from build123d import *

# Parameters (mm, degrees)
SKETCH_W      = 80
SKETCH_H      = 150
PAD_DEPTH     = 2
FILLET_R      = 10
SKETCH001_R   = 19.147904
SKETCH001_R_2 = 1.5
POCKET_DEPTH  = 5


with BuildPart() as part:
    # Sketch → Pad (new body)
    with BuildSketch(Plane.XZ):
        with Locations((40, 75)):
            Rectangle(SKETCH_W, SKETCH_H)
    extrude(amount=PAD_DEPTH)

    # Fillet
    fillet_edges = [part.edges().sort_by_distance(p)[0] for p in [
        (0, -1, 0),
        (0, -1, 150),
        (80, -1, 150),
        (80, -1, 0),
    ]]
    fillet(fillet_edges, radius=FILLET_R)

    # Sketch001 (on Face2 of Fillet) → Pocket (cut)
    with BuildSketch(Plane(origin=(0, 0, 0), x_dir=(1, 0, 0), z_dir=(0, 1, 0))):
        with Locations((40, -40)):
            Circle(SKETCH001_R)
        with Locations((21, -21)):
            Circle(SKETCH001_R_2)
        with Locations((59, -21)):
            Circle(SKETCH001_R_2)
        with Locations((59, -59)):
            Circle(SKETCH001_R_2)
        with Locations((21, -59)):
            Circle(SKETCH001_R_2)
    extrude(amount=-POCKET_DEPTH, mode=Mode.SUBTRACT)


solid = part.part
Read the model definition and answer for the solid it produces. Units are mm, in the model's axes. Round coordinates to 2 decimals unless told otherwise and drop trailing zeros. Write each loop counter-clockwise with the first axis right and the second up, starting at its lowest first coordinate (ties: lowest second). Pieces come first, ordered by that corner, then holes. Notation, with made-up numbers: (-16.5, 53) - (37.5, 53) arc R28 cw to (37.5, 92) - close; hole circle Ø3 at (52.5, 64). An arc over 180 degrees is marked (long way). One line per question, with ' | ' between items. Start each with the question number.
1. For a pull along X with two mould halves and no side action, classify faces 1 (the face through (60.43, -0.99, 58.55)), 2 (the face through (76.99, -1.01, 2.85)), 3 (the face through (2.85, -1.01, 146.99)) as +X half, -X half, draft (parallel to the pull), parting line (faces both ways), or undercut.
2. Section C-C (y = -1.5) is taken. Determine the outline of the cut face in (x, z), and give its area (3 significant figures).
3. Section B-B (z = 40) is taken. Determine the outline of the cut face in (x, y), and give its area (3 significant figures).
4. Section A-A (x = 40) is taken. Determine the outline of the cut face in (y, z).
5. Find the intervals of material crossed by probe 1 along X at (y, z) = (-0.75, 40); probe 2 along X at (y, z) = (-0.75, 48.5); probe 3 along Z at (x, y) = (38, -0.9), in increasing order. Write a range as [from, to].
6. This flat-tipped pin is pushed along its axis until it touches: pin 1 (2.5 mm diameter, centred on x = 21, z = 21, fed in from +Y). Where does it stop, or does it pass through?
Filled in:
1) face 1: undercut | face 2: +X half | face 3: -X half
2) outline: (0, 10) arc R10 ccw to (10, 0) - (70, 0) arc R10 ccw to (80, 10) - (80, 140) arc R10 ccw to (70, 150) - (10, 150) arc R10 ccw to (0, 140) - close; hole circle Ø3 at (21, 21); hole circle Ø3 at (21, 59); hole circle Ø38.3 at (40, 40); hole circle Ø3 at (59, 21); hole circle Ø3 at (59, 59) | area: 10,700 mm²
3) outline: (0, -2) - (20.85, -2) - (20.85, 0) - (0, 0) - close; (59.15, -2) - (80, -2) - (80, 0) - (59.15, 0) - close | area: 83.4 mm²
4) outline: (-2, 0) - (0, 0) - (0, 20.85) - (-2, 20.85) - close; (-2, 59.15) - (0, 59.15) - (0, 150) - (-2, 150) - close
5) probe 1: [0, 20.85], [59.15, 80] | probe 2: [0, 22.84], [57.16, 80] | probe 3: [0, 20.96], [59.04, 150]
6) pin 1: through
